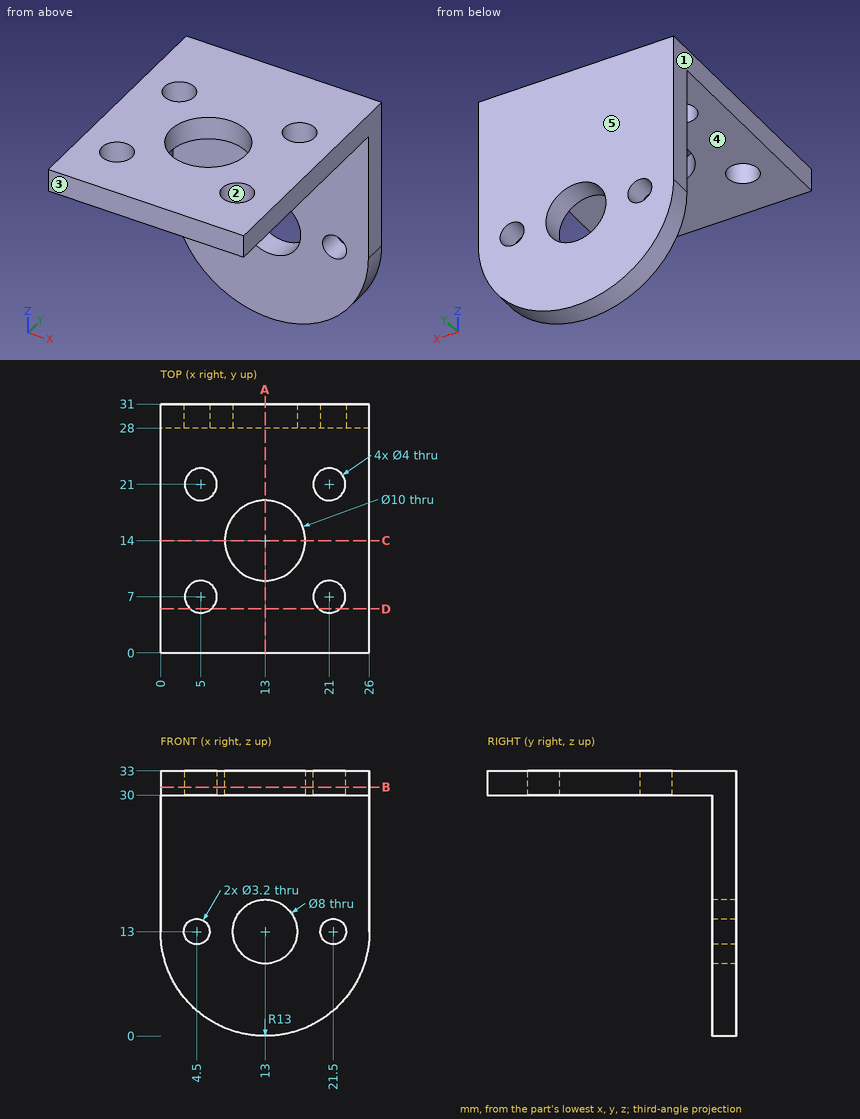
The figure shows three views and two pictorial views of one solid part (mm, origin at its lowest corner). Answer the questions. A direction names the side the tool comes from. Coordinates: 2 decimals unless noted, no trailing zeros. Loops run counter-clockwise (first coordinate to the right, second up) from the corner with the lowest first, then second, coordinate; pieces in that order, holes last. Notation, with made-up numbers: (35, 34.25) - (57, 34.25) arc R21 cw to (57, 61.25) - close; hole circle Ø8 at (-27, -2.5). An arc over 180 degrees is marked (long way). Write item = value, one per line.
1) Find the intervals of material crossed by line 1 along Y through (x, z) = (21, 31.6); line 2 along Z through (x, y) = (16, 20.5); line 3 along Y through (x, z) = (16.5, 4.5), in increasing order.
Responses:
line_1 = 0 to 5, 9 to 19, 23 to 31
line_2 = 30 to 33
line_3 = 28 to 31
2) Section C-C (y = 14) is taken. Determine the outline of the cut face in (x, z).
Responses:
outline = (0, 30) - (8, 30) - (8, 33) - (0, 33) - close; (18, 30) - (26, 30) - (26, 33) - (18, 33) - close
3) Section B-B (z = 31) is taken. Determine the outline of the cut face in (x, y), plus the area to 3 significant figures.
Responses:
outline = (0, 0) - (26, 0) - (26, 31) - (0, 31) - close; hole circle Ø4 at (5, 7); hole circle Ø4 at (5, 21); hole circle Ø10 at (13, 14); hole circle Ø4 at (21, 7); hole circle Ø4 at (21, 21)
area = 677 mm^2
4) Section A-A (x = 13) is taken. Determine the outline of the cut face in (y, z), plus the area to 3 significant figures.
Responses:
outline = (0, 30) - (9, 30) - (9, 33) - (0, 33) - close; (19, 30) - (28, 30) - (28, 17) - (31, 17) - (31, 33) - (19, 33) - close; (28, 0) - (31, 0) - (31, 9) - (28, 9) - close
area = 129 mm^2
5) Each of these flat-tipped pins is pushed along its axis until it touches: P1, Ø8, axis at x = 13, y = 14, coming from the -Z side; P2, Ø5, axis at x = 9.5, y = 8.5, coming from the -Z side; P3, Ø13, axis at x = 17, z = 13, coming from the -Y side. Where does it stop, or does it pass through?
Responses:
P1 = through
P2 = 30
P3 = 28
6) Section D-D (y = 5.5) is taken. Determine the outline of the cut face in (x, z).
Responses:
outline = (0, 30) - (3.68, 30) - (3.68, 33) - (0, 33) - close; (6.32, 30) - (19.68, 30) - (19.68, 33) - (6.32, 33) - close; (22.32, 30) - (26, 30) - (26, 33) - (22.32, 33) - close
7) Which of the six approach directions +Z, -Z, +X, -X, +Y, -Y give full straight-line access (tool end or side, diameter ignored) to the marked faces 4 and 5?
Responses:
face_4 = -Z, +X, -X, -Y
face_5 = +Z, -Z, +X, -X, +Y
8) Determine the mould class of the marked faces 1, 2 and 3 for opening direction X: pulls with the +X half, pulls with the -X half, needs draft (parallel to the pull), parting line crosses it, or undercut.
Responses:
face_1 = pulls with the -X half
face_2 = undercut
face_3 = needs draft
